Source: CAD feature listing. Evaluate the final solid. Frame: model axes, mm. A direction names the side the tool comes from. Coordinates: 2 decimals unless noted, no trailing zeros. Order: outer loops, then holes, each group sorted by start corner. A loop starts at its lowest first (then second) coordinate and runs counter-clockwise, first axis right, second up. Notation, with made-up numbers: (25, 31) -> (59, 31) arc R20 cw to (59, 47) -> close; hole circle Ø6 at (34, 0.25). An arc over 180 degrees is marked (long way). Put each result on its own line as item: value.
from build123d import *

# Parameters (mm, degrees)
F0_W     = 229
F0_H     = 149
F1_DEPTH = 10
F2_DEPTH = 5
F3_R     = 19


with BuildPart() as f1:
    # F0 (on Top) → F1 (new body)
    with BuildSketch(Plane.XY):
        Polygon((30, 0), (0, 0), (0, -35), (30.5, -35), (30.5, -43), (30.5, -184), (30.5, -188.999996), (35.5, -188.999996), (264.5, -188.999996), (269.5, -188.999996), (269.5, -184), (269.5, -43), (269.5, -35), (300, -35), (300, 0), (270, 0), (270, -10), (150, -10), (30, -10), align=None)
        with Locations((150, -109.5)):
            Rectangle(F0_W, F0_H, mode=Mode.SUBTRACT)
    extrude(amount=F1_DEPTH)

    # F0 (on Top) → F2 (join)
    with BuildSketch(Plane.XY):
        Polygon((30.5, -43), (0, -43), (0, -219), (300, -219), (300, -43), (269.5, -43), (269.5, -184), (269.5, -188.999996), (264.5, -188.999996), (35.5, -188.999996), (30.5, -188.999996), (30.5, -184), align=None)
    extrude(amount=F2_DEPTH)

    # F3
    f3_edges = [f1.edges().sort_by_distance(p)[0] for p in [
        (0, 0, 5),
        (300, 0, 5),
        (300, -219, 2.5),
        (0, -219, 2.5),
    ]]
    fillet(f3_edges, radius=F3_R)


solid = f1.part
1. Cut plane B-B on z = 3.25. Output: boundary loops of the cut face in (x, y).
Numbers:
outline: (0, -200) arc R19 ccw to (19, -219) -> (281, -219) arc R19 ccw to (300, -200) -> (300, -43) -> (269.5, -43) -> (269.5, -35) -> (300, -35) -> (300, -19) arc R19 ccw to (281, 0) -> (270, 0) -> (270, -10) -> (30, -10) -> (30, 0) -> (19, 0) arc R19 ccw to (0, -19) -> (0, -35) -> (30.5, -35) -> (30.5, -43) -> (0, -43) -> close; hole (35.5, -184) -> (264.5, -184) -> (264.5, -35) -> (35.5, -35) -> close
2. Cut plane C-C on y = -165. Output: boundary loops of the cut face in (x, z), plus the area to 3 significant figures.
Numbers:
outline: (0, 0) -> (35.5, 0) -> (35.5, 10) -> (30.5, 10) -> (30.5, 5) -> (0, 5) -> close; (264.5, 0) -> (300, 0) -> (300, 5) -> (269.5, 5) -> (269.5, 10) -> (264.5, 10) -> close
area: 405 mm2
3. Cut plane D-D on y = -204.5. Output: boundary loops of the cut face in (x, z), plus the area to 3 significant figures.
Numbers:
outline: (0.54, 0) -> (299.46, 0) -> (299.46, 5) -> (0.54, 5) -> close
area: 1,490 mm2
4. First-contact query: pin 1 (1.5 mm diameter, centred on x = 113, z = 6.5, fed in from -Y); pin 2 (4 mm diameter, centred on x = 76, z = 7, fed in from +Y); pin 3 (5 mm diameter, centred on x = 14.5, z = 4, fed in from -Y). Flat tips, straight axial feed; report the tip coordinate or a pass-through.
Numbers:
pin 1: stops at y = -189
pin 2: stops at y = -10
pin 3: stops at y = -218.89
5. Cut plane A-A on x = 97. Output: boundary loops of the cut face in (y, z).
Numbers:
outline: (-219, 0) -> (-184, 0) -> (-184, 10) -> (-189, 10) -> (-189, 5) -> (-219, 5) -> close; (-35, 0) -> (-10, 0) -> (-10, 10) -> (-35, 10) -> close
6. Set-up query: faces 1 (the flat face through (270, -5, 5)), 2 (the flat face through (285, -35, 5)), 3 (the flat face through (148, -35, 5)). Return all of +Z, -Z, +X, -X, +Y, -Y with unobstructed straight access to the full face (end or side cutting, diameter ignored); none if empty.
Numbers:
face 1: +Z, -Z, +Y
face 2: +Z, -Z, +X
face 3: +Z, -Z
7. Pull-direction query (X, two-part tool) for faces 4 (the cylindrical face through (5.71, -5.42, 5.07)), 5 (the flat face through (30, -5, 5)), 6 (the flat face through (276, 0, 5)); classes: pulls with the +X half, pulls with the -X half, needs draft (parallel to the pull), parting line crosses it, or undercut.
Numbers:
face 4: pulls with the -X half
face 5: undercut
face 6: needs draft
8. Ray query, line 1 along Y through (x, z) = (76.5, 9.75); line 2 along Y through (x, z) = (233, 4); line 3 along X through (y, z) = (-57, 6). Return the intervals inside material, ascending.
Numbers:
line 1: y = -189 to -184, -35 to -10
line 2: y = -219 to -184, -35 to -10
line 3: x = 30.5 to 35.5, 264.5 to 269.5
